```python
from build123d import *

# Parameters (mm, degrees)
SKETCH1_R           = 2.6035
BOSS_EXTRUDE1_DEPTH = 80


with BuildPart() as part:
    # Sketch1 → Boss-Extrude1 (new body, symmetric)
    with BuildSketch(Plane.XY):
        with BuildLine():
            Line((-7.179650497, -8.645192506), (-3.952270251, -5.423690499))
            ThreePointArc((-3.952270251, -5.423690499), (-2.922936451, -4.736929036), (-1.709253557, -4.4958))
            Line((-1.709253557, -4.4958), (1.709253557, -4.4958))
            ThreePointArc((1.709253557, -4.4958), (2.922936451, -4.736929036), (3.952270251, -5.423690499))
            Line((3.952270251, -5.423690499), (7.179650497, -8.645192506))
            ThreePointArc((7.179650497, -8.645192506), (7.41473083, -9.822813117), (6.416408329, -10.4902))
            Line((6.416408329, -10.4902), (4.287512407, -10.4902))
            ThreePointArc((4.287512407, -10.4902), (3.54574862, -10.79744862), (3.2385, -11.539212407))
            Line((3.2385, -11.539212407), (3.2385, -11.650987593))
            ThreePointArc((3.2385, -11.650987593), (3.54574862, -12.39275138), (4.287512407, -12.7))
            Line((4.287512407, -12.7), (5.317126718, -12.7))
            ThreePointArc((5.317126718, -12.7), (5.825126718, -12.192), (6.333126718, -12.7))
            Line((6.333126718, -12.7), (9.550443118, -12.7))
            ThreePointArc((9.550443118, -12.7), (10.058366869, -12.192000006), (10.566443095, -12.699847501))
            ThreePointArc((10.566443095, -12.699847501), (12.082537762, -12.08250727), (12.699846982, -10.566399977))
            ThreePointArc((12.699846982, -10.566399977), (12.192000006, -10.058323491), (12.7, -9.5504))
            Line((12.7, -9.5504), (12.7, -6.3330836))
            ThreePointArc((12.7, -6.3330836), (12.192, -5.8250836), (12.7, -5.3170836))
            Line((12.7, -5.3170836), (12.7, -4.287469289))
            ThreePointArc((12.7, -4.287469289), (12.39275138, -3.545705502), (11.650987593, -3.238456882))
            Line((11.650987593, -3.238456882), (11.539212407, -3.238456882))
            ThreePointArc((11.539212407, -3.238456882), (10.79744862, -3.545705502), (10.4902, -4.287469289))
            Line((10.4902, -4.287469289), (10.4902, -6.402089023))
            ThreePointArc((10.4902, -6.402089023), (9.856505071, -7.351067942), (8.737131347, -7.129408934))
            Line((8.737131347, -7.129408934), (5.441005833, -3.840816462))
            ThreePointArc((5.441005833, -3.840816462), (4.750877967, -2.809883091), (4.5085, -1.593185507))
            Line((4.5085, -1.593185507), (4.5085, 1.593185507))
            ThreePointArc((4.5085, 1.593185507), (4.750877967, 2.809883091), (5.441005833, 3.840816462))
            Line((5.441005833, 3.840816462), (8.737131347, 7.129408934))
            ThreePointArc((8.737131347, 7.129408934), (9.856505071, 7.351067942), (10.4902, 6.402089023))
            Line((10.4902, 6.402089023), (10.4902, 4.287469289))
            ThreePointArc((10.4902, 4.287469289), (10.79744862, 3.545705502), (11.539212407, 3.238456882))
            Line((11.539212407, 3.238456882), (11.650987593, 3.238456882))
            ThreePointArc((11.650987593, 3.238456882), (12.39275138, 3.545705502), (12.7, 4.287469289))
            Line((12.7, 4.287469289), (12.7, 5.3170836))
            ThreePointArc((12.7, 5.3170836), (12.192, 5.8250836), (12.7, 6.3330836))
            Line((12.7, 6.3330836), (12.7, 9.5504))
            ThreePointArc((12.7, 9.5504), (12.192000006, 10.058323491), (12.699846982, 10.566399977))
            ThreePointArc((12.699846982, 10.566399977), (12.082537762, 12.08250727), (10.566443095, 12.699847501))
            ThreePointArc((10.566443095, 12.699847501), (10.058366869, 12.192000006), (9.550443118, 12.7))
            Line((9.550443118, 12.7), (6.333126718, 12.7))
            ThreePointArc((6.333126718, 12.7), (5.825126718, 12.192), (5.317126718, 12.7))
            Line((5.317126718, 12.7), (4.287512407, 12.7))
            ThreePointArc((4.287512407, 12.7), (3.54574862, 12.39275138), (3.2385, 11.650987593))
            Line((3.2385, 11.650987593), (3.2385, 11.539212407))
            ThreePointArc((3.2385, 11.539212407), (3.54574862, 10.79744862), (4.287512407, 10.4902))
            Line((4.287512407, 10.4902), (6.476788598, 10.4902))
            ThreePointArc((6.476788598, 10.4902), (7.432222385, 9.85140422), (7.207036008, 8.724370562))
            Line((7.207036008, 8.724370562), (3.898272566, 5.423169045))
            ThreePointArc((3.898272566, 5.423169045), (2.869120213, 4.736787962), (1.655778399, 4.4958))
            Line((1.655778399, 4.4958), (-1.655778399, 4.4958))
            ThreePointArc((-1.655778399, 4.4958), (-2.869120213, 4.736787962), (-3.898272566, 5.423169045))
            Line((-3.898272566, 5.423169045), (-7.207036008, 8.724370562))
            ThreePointArc((-7.207036008, 8.724370562), (-7.432222385, 9.85140422), (-6.476788598, 10.4902))
            Line((-6.476788598, 10.4902), (-4.287512407, 10.4902))
            ThreePointArc((-4.287512407, 10.4902), (-3.54574862, 10.79744862), (-3.2385, 11.539212407))
            Line((-3.2385, 11.539212407), (-3.2385, 11.650987593))
            ThreePointArc((-3.2385, 11.650987593), (-3.54574862, 12.39275138), (-4.287512407, 12.7))
            Line((-4.287512407, 12.7), (-5.317126718, 12.7))
            ThreePointArc((-5.317126718, 12.7), (-5.825126718, 12.192), (-6.333126718, 12.7))
            Line((-6.333126718, 12.7), (-9.550443118, 12.7))
            ThreePointArc((-9.550443118, 12.7), (-10.058366869, 12.192000006), (-10.566443095, 12.699847501))
            ThreePointArc((-10.566443095, 12.699847501), (-12.082537762, 12.08250727), (-12.699846982, 10.566399977))
            ThreePointArc((-12.699846982, 10.566399977), (-12.192000006, 10.058323491), (-12.7, 9.5504))
            Line((-12.7, 9.5504), (-12.7, 6.3330836))
            ThreePointArc((-12.7, 6.3330836), (-12.192, 5.8250836), (-12.7, 5.3170836))
            Line((-12.7, 5.3170836), (-12.7, 4.287469289))
            ThreePointArc((-12.7, 4.287469289), (-12.39275138, 3.545705502), (-11.650987593, 3.238456882))
            Line((-11.650987593, 3.238456882), (-11.539212407, 3.238456882))
            ThreePointArc((-11.539212407, 3.238456882), (-10.79744862, 3.545705502), (-10.4902, 4.287469289))
            Line((-10.4902, 4.287469289), (-10.4902, 6.402089023))
            ThreePointArc((-10.4902, 6.402089023), (-9.856505071, 7.351067942), (-8.737131347, 7.129408934))
            Line((-8.737131347, 7.129408934), (-5.441005833, 3.840816462))
            ThreePointArc((-5.441005833, 3.840816462), (-4.750877967, 2.809883091), (-4.5085, 1.593185507))
            Line((-4.5085, 1.593185507), (-4.5085, -1.593185507))
            ThreePointArc((-4.5085, -1.593185507), (-4.750877967, -2.809883091), (-5.441005833, -3.840816462))
            Line((-5.441005833, -3.840816462), (-8.737131347, -7.129408934))
            ThreePointArc((-8.737131347, -7.129408934), (-9.856505071, -7.351067942), (-10.4902, -6.402089023))
            Line((-10.4902, -6.402089023), (-10.4902, -4.287469289))
            ThreePointArc((-10.4902, -4.287469289), (-10.79744862, -3.545705502), (-11.539212407, -3.238456882))
            Line((-11.539212407, -3.238456882), (-11.650987593, -3.238456882))
            ThreePointArc((-11.650987593, -3.238456882), (-12.39275138, -3.545705502), (-12.7, -4.287469289))
            Line((-12.7, -4.287469289), (-12.7, -5.3170836))
            ThreePointArc((-12.7, -5.3170836), (-12.192, -5.8250836), (-12.7, -6.3330836))
            Line((-12.7, -6.3330836), (-12.7, -9.5504))
            ThreePointArc((-12.7, -9.5504), (-12.192000006, -10.058323491), (-12.699846982, -10.566399977))
            ThreePointArc((-12.699846982, -10.566399977), (-12.082537762, -12.08250727), (-10.566443095, -12.699847501))
            ThreePointArc((-10.566443095, -12.699847501), (-10.058366869, -12.192000006), (-9.550443118, -12.7))
            Line((-9.550443118, -12.7), (-6.333126718, -12.7))
            ThreePointArc((-6.333126718, -12.7), (-5.825126718, -12.192), (-5.317126718, -12.7))
            Line((-5.317126718, -12.7), (-4.287512407, -12.7))
            ThreePointArc((-4.287512407, -12.7), (-3.54574862, -12.39275138), (-3.2385, -11.650987593))
            Line((-3.2385, -11.650987593), (-3.2385, -11.539212407))
            ThreePointArc((-3.2385, -11.539212407), (-3.54574862, -10.79744862), (-4.287512407, -10.4902))
            Line((-4.287512407, -10.4902), (-6.416408329, -10.4902))
            ThreePointArc((-6.416408329, -10.4902), (-7.41473083, -9.822813117), (-7.179650497, -8.645192506))
        make_face()
        Circle(SKETCH1_R, mode=Mode.SUBTRACT)
    extrude(amount=BOSS_EXTRUDE1_DEPTH, both=True)


solid = part.part
```
CAD build for the part. Positions are in the model's coordinates, mm. A direction names the side the tool comes from. Coordinates: 2 decimals unless noted, no trailing zeros. Order: outer loops, then holes, each group sorted by start corner. A loop starts at its lowest first (then second) coordinate and runs counter-clockwise, first axis right, second up.
(1) Mould opens along Y. For faces 4 (the face through (5.58, 7.1, 1.12)), 5 (the face through (3, 0, -80)), 6 (the face through (2.483, 0.782, -1.12)), 7 (the face through (8, 12.7, 1)) say: released by +Y, released by -Y, zero draft, split by the parting line, or undercut.
Solution:
face 4: undercut
face 5: zero draft
face 6: undercut
face 7: released by +Y
(2) Saw through at B-B, the plane y = 0. Write the cut outline in (x, z).
Solution:
outline: (-4.51, -80) - (-2.6, -80) - (-2.6, 80) - (-4.51, 80) - close; (2.6, -80) - (4.51, -80) - (4.51, 80) - (2.6, 80) - close
(3) Saw through at A-A, the plane x = 0. Write the cut outline in (y, z), and give its area (3 significant figures).
Solution:
outline: (-4.5, -80) - (-2.6, -80) - (-2.6, 80) - (-4.5, 80) - close; (2.6, -80) - (4.5, -80) - (4.5, 80) - (2.6, 80) - close
area: 606 mm2
(4) Which spindle directions (+Z, -Z, +X, -X, +Y, -Y) get a long thin tool onto all of the face, cutting with end or side? Do faces 1 (the face through (-5.59, -7.06, 1.12)), 2 (the face through (-4.508, 0, 1)), 3 (the face through (0, 4.496, 1)). Say none if no direction does.
Solution:
face 1: +Z, -Z
face 2: +Z, -Z, -X
face 3: +Z, -Z, +Y
(5) Drill centre lines: L1, parallel to Y at x = 0, z = 35.5; L2, parallel to X at y = 7, z = -69.5; L3, parallel to X at y = -5, z = 35.5. Where is each one in solid material? Low to high.
Solution:
L1: y = -4.5 to -2.6, 2.6 to 4.5
L2: x = -12.7 to -10.3, -8.61 to -5.48, 5.48 to 8.61, 10.3 to 12.7
L3: x = -12.7 to -10.49, -6.6 to -3.43, 3.43 to 6.6, 10.49 to 12.7
(6) Pin check, flat tips, straight feed: pin 1 Ø1.5 at (y, z) = (0.5, 57.5) entering from +X; pin 2 Ø5 at (x, y) = (-8, -2) entering from +Z; pin 3 Ø1.1 at (x, z) = (5.5, -30) entering from -Y; pin 4 Ø1.7 at (x, z) = (-0.5, 11) entering from -Y. Stop position of each tip, or through.
Solution:
pin 1: stops at x = 4.51
pin 2: passes through
pin 3: stops at y = -12.7
pin 4: stops at y = -4.5
